from build123d import *

# Parameters (mm, degrees)
F0_R           = 11.4
F1_DEPTH       = 0.01
F2_R           = 11.4
F2_R_2         = 9
F3_DEPTH       = 20
F5_DEPTH       = 10
F5_DEPTH_BACK  = 10
F7_DEPTH       = 10
F7_DEPTH_BACK  = 10
F9_DEPTH       = 11.401
F9_DEPTH_BACK  = 11.401
F10_R          = 2.6
F11_DEPTH      = 11.4010001
F11_DEPTH_BACK = 11.4010001
F12_R          = 9
F13_DEPTH      = 10
F14_R          = 27
F15_DEPTH      = 2.5
F16_R          = 2.75
F17_DEPTH      = 25
F18_R          = 0.75
F19_DEPTH      = 25


with BuildPart() as f1:
    # F0 (on Top) → F1 (new body)
    with BuildSketch(Plane.XY):
        Circle(F0_R)
    extrude(amount=F1_DEPTH)

    # F2 (on face) → F3 (join)
    with BuildSketch(Plane.XY.offset(0.01)):
        Circle(F2_R)
        Circle(F2_R_2, mode=Mode.SUBTRACT)
    extrude(amount=F3_DEPTH)

    # F4 (on Right) → F5 (cut, two sides)
    with BuildSketch(Plane.YZ) as f5_sk:
        Polygon((-2.3094010768, 6), (2.3094010768, 6), (4.6188021535, 10), (2.3094010768, 14), (-2.3094010768, 14), (-4.6188021535, 10), align=None)
    extrude(amount=F5_DEPTH, mode=Mode.SUBTRACT)
    extrude(f5_sk.sketch, amount=-F5_DEPTH_BACK, mode=Mode.SUBTRACT)

    # F6 (on Front) → F7 (cut, two sides)
    with BuildSketch(Plane.XZ) as f7_sk:
        Polygon((-2.3094010768, 6), (2.3094010768, 6), (4.6188021535, 10), (2.3094010768, 14), (-2.3094010768, 14), (-4.6188021535, 10), align=None)
    extrude(amount=F7_DEPTH, mode=Mode.SUBTRACT)
    extrude(f7_sk.sketch, amount=-F7_DEPTH_BACK, mode=Mode.SUBTRACT)

    # F8 (on Right) → F9 (cut, two sides)
    with BuildSketch(Plane.YZ) as f9_sk:
        with BuildLine():
            ThreePointArc((0, 12.6), (-2.6, 10), (0, 7.4))
            Line((0, 7.4), (0, 12.6))
        make_face()
        with BuildLine():
            Line((0, 12.6), (0, 7.4))
            ThreePointArc((0, 7.4), (1.8384776311, 8.1615223689), (2.6, 10))
            ThreePointArc((2.6, 10), (1.8384776311, 11.8384776311), (0, 12.6))
        make_face()
    extrude(amount=-F9_DEPTH, mode=Mode.SUBTRACT)
    extrude(f9_sk.sketch, amount=F9_DEPTH_BACK, mode=Mode.SUBTRACT)

    # F10 (on Front) → F11 (cut, two sides)
    with BuildSketch(Plane.XZ) as f11_sk:
        with Locations((0, 10)):
            Circle(F10_R)
    extrude(amount=F11_DEPTH, mode=Mode.SUBTRACT)
    extrude(f11_sk.sketch, amount=-F11_DEPTH_BACK, mode=Mode.SUBTRACT)

    # F12 (on face) → F13 (cut)
    with BuildSketch(Plane.XY.offset(0.01)):
        Circle(F12_R)
    extrude(amount=-F13_DEPTH, mode=Mode.SUBTRACT)

    # F14 (on face) → F15 (join)
    with BuildSketch(Plane.XY.offset(20.01)):
        Circle(F14_R)
    extrude(amount=F15_DEPTH)

    # F16 (on face) → F17 (cut)
    with BuildSketch(Plane.XY.offset(22.51)):
        with Locations((2.5, 0)):
            Circle(F16_R)
    extrude(amount=-F17_DEPTH, mode=Mode.SUBTRACT)

    # F18 (on face) → F19 (cut)
    with BuildSketch(Plane.XY.offset(22.51)):
        with Locations((-16, -16)):
            Circle(F18_R)
        with Locations((16, -16)):
            Circle(F18_R)
        with Locations((-16, 16)):
            Circle(F18_R)
        with Locations((16, 16)):
            Circle(F18_R)
    extrude(amount=-F19_DEPTH, mode=Mode.SUBTRACT)


solid = f1.part
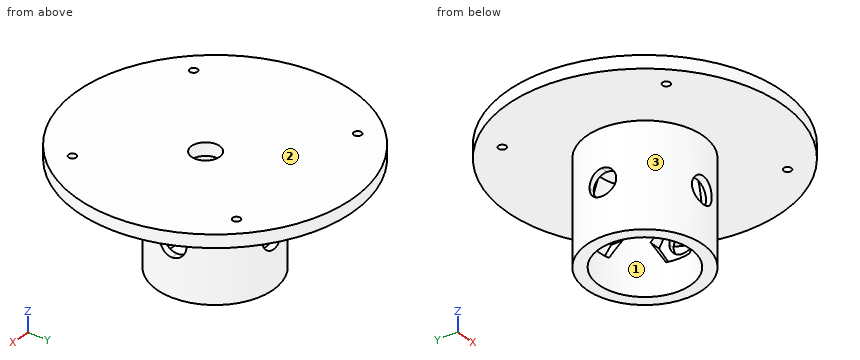
Here's how the part is built. I have some questions about the finished solid (model axes, mm). Face numbers are marked on the shaded views. Give positions to 0.01 mm unless a question says otherwise; leave off trailing zeros. Order: outer loops, then holes, each group sorted by start corner. A loop starts at its lowest first (then second) coordinate and runs counter-clockwise, first axis right, second up. Notation, with made-up numbers: (86.25, 68) -> (127.25, 68) arc R10 ccw to (127.25, 83) -> close; hole circle Ø2 at (-16, 26). An arc over 180 degrees is marked (long way). Use a Markdown table: item, result. Add a question column.
Item 1: If we mould it in two halves opening along X, with no side actions, what happens to the marked faces 1, 2 and 3? For each: pulls with the +X half, pulls with the -X half, needs draft (parallel to the pull), parting line crosses it, or undercut.
Item 2: Imagine slicing it at D-D on z = 18.75. Please give me the cut outline in (x, y), plus the area to 3 significant figures.
Item 3: Imagine slicing it at B-B on y = -16. Please give me the cut outline in (x, z), plus the area to 3 significant figures.
Item 4: Imagine slicing it at A-A on z = 11.75. Give the number of separate pieces and of enclosed holes in the cut face, plus the area to 3 significant figures.
Item 5: Will these pins go through, and if not, where does the flat tip stop? pin 1 (10 mm diameter, centred on y = -4.5, z = 20, fed in from -X); pin 2 (6 mm diameter, centred on x = 0, z = 10, fed in from +Y); pin 3 (3 mm diameter, centred on x = 5.5, y = 20, fed in from -Z); pin 4 (3 mm diameter, centred on x = 11, z = 19, fed in from -Y).
Item 6: I need wall thicknesses on line 1 (Y direction, x = 16, z = 21.3); line 2 (Y direction, x = 0, z = 7.25); line 3 (Z direction, x = -19.5, y = 12.5). Which ranges of each line are inside material? Lowest first, please.
Data:
| question | item | result |
|---|---|---|
| 1 | face 1 | undercut |
| 1 | face 2 | needs draft |
| 1 | face 3 | parting line crosses it |
| 2 | outline | circle Ø22.8 at (0, 0); hole circle Ø18 at (0, 0) |
| 2 | area | 154 mm² |
| 3 | outline | (-21.75, 20.01) -> (-16.75, 20.01) -> (-16.75, 22.51) -> (-21.75, 22.51) -> close; (-15.25, 20.01) -> (15.25, 20.01) -> (15.25, 22.51) -> (-15.25, 22.51) -> close; (16.75, 20.01) -> (21.75, 20.01) -> (21.75, 22.51) -> (16.75, 22.51) -> close |
| 3 | area | 101 mm² |
| 4 | separate pieces | 4 |
| 4 | enclosed holes | 0 |
| 4 | area | 97.1 mm² |
| 5 | pin 1 | stops at x = -27 |
| 5 | pin 2 | stops at y = 11.4 |
| 5 | pin 3 | stops at z = 20.01 |
| 5 | pin 4 | stops at y = -25.12 |
| 6 | line 1 | y = -21.75 to -16.75, -15.25 to 15.25, 16.75 to 21.75 |
| 6 | line 2 | y = -11.4 to -10, 10 to 11.4 |
| 6 | line 3 | z = 20.01 to 22.51 |
